Build history of the part. All positions in model axes, mm. Give positions to 0.01 mm unless a question says otherwise; leave off trailing zeros. Order: outer loops, then holes, each group sorted by start corner. A loop starts at its lowest first (then second) coordinate and runs counter-clockwise, first axis right, second up. Notation, with made-up numbers: (-36, 8) - (8, 8) arc R18 cw to (8, 24) - close; hole circle Ø7 at (-30.5, 39.5). An arc over 180 degrees is marked (long way). Use a Markdown table: item, result.
from build123d import *

# Parameters (mm, degrees)
F1_DEPTH = 2.15
F3_DEPTH = 3.1
F5_DEPTH = 0.8
F9_DEPTH = 1.4


with BuildPart() as f1:
    # F0 (on Top) → F1 (new body)
    with BuildSketch(Plane.XY):
        Polygon((-50.2594385356, -11.2599956296), (0, -11.2599956296), (0, 6.3900043704), (-47.2094385356, 6.3900043704), (-47.2094385356, 1.7900043704), (-47.9594385356, 1.7900043704), (-47.9594385356, 10.5400043704), (-50.2594385356, 10.5400043704), align=None)
        Polygon((0, 6.3900043704), (0, -11.2599956296), (50.2594385356, -11.2599956296), (50.2594385356, 10.5400043704), (47.9594385356, 10.5400043704), (47.9594385356, 1.7900043704), (47.2094385356, 1.7900043704), (47.2094385356, 6.3900043704), align=None)
    extrude(amount=F1_DEPTH)

    # F2 (on face) → F3 (join)
    with BuildSketch(Plane.XY.offset(2.15)):
        Polygon((-47.9594385356, -9.0099956296), (-47.9594385356, 1.7900043704), (-47.9594385356, 10.5400043704), (-50.2594385356, 10.5400043704), (-50.2594385356, -11.2599956296), (50.2594385356, -11.2599956296), (50.2594385356, 10.5400043704), (47.9594385356, 10.5400043704), (47.9594385356, 1.7900043704), (47.9594385356, -9.0099956296), (0, -9.0099956296), align=None)
    extrude(amount=F3_DEPTH)

    # F4 (on face) → F5 (cut)
    with BuildSketch(Plane.XY.offset(5.25)):
        with BuildLine():
            Line((-49.6594385356, -9.0099956296), (-49.6594385356, 7.0900043704))
            Line((-49.6594385356, 7.0900043704), (-47.9594385356, 7.0900043704))
            Line((-47.9594385356, 7.0900043704), (-47.9594385356, 10.5400043704))
            Line((-47.9594385356, 10.5400043704), (-50.2594385356, 10.5400043704))
            Line((-50.2594385356, 10.5400043704), (-50.2594385356, -11.2599956296))
            Line((-50.2594385356, -11.2599956296), (50.2594385356, -11.2599956296))
            Line((50.2594385356, -11.2599956296), (50.2594385356, 10.5400043704))
            Line((50.2594385356, 10.5400043704), (47.9594385356, 10.5400043704))
            Line((47.9594385356, 10.5400043704), (47.9594385356, 7.0900043704))
            Line((47.9594385356, 7.0900043704), (49.6594385356, 7.0900043704))
            Line((49.6594385356, 7.0900043704), (49.6594385356, -9.0099956296))
            ThreePointArc((49.6594385356, -9.0099956296), (49.1615200636, -10.2120771576), (47.9594385356, -10.7099956296))
            Line((47.9594385356, -10.7099956296), (0, -10.7099956296))
            Line((0, -10.7099956296), (-47.9594385356, -10.7099956296))
            ThreePointArc((-47.9594385356, -10.7099956296), (-49.1615200636, -10.2120771576), (-49.6594385356, -9.0099956296))
        make_face()
    extrude(amount=-F5_DEPTH, mode=Mode.SUBTRACT)

    # F8 (on plane+point) → F9 (join)
    with BuildSketch(Plane(origin=(0, -1.5099956296, 0), x_dir=(-1, 0, 0), z_dir=(0, 1, 0))):
        Polygon((47.2594385356, 6.1), (39.3594385356, 2.15), (47.9594385356, 2.15), (47.9594385356, 5.25), (47.2594385356, 5.25), align=None)
    extrude(amount=F9_DEPTH)

    # F10: F1 across plane


with BuildPart() as f1_1:
    add(f1.part)
    add(f1.part.mirror(Plane.YZ))


solid = f1_1.part
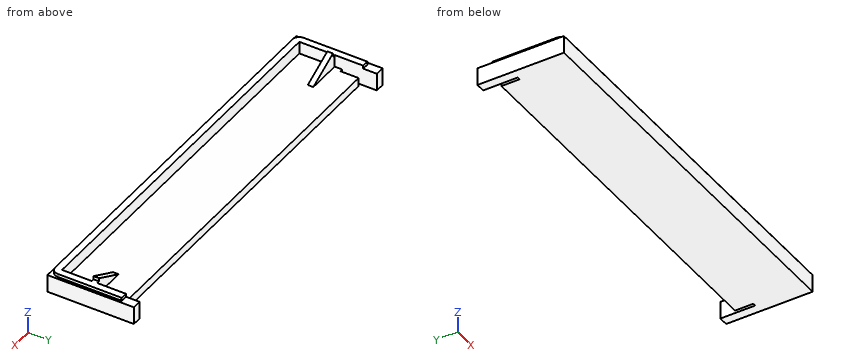
1) Slice it at D-D (y = -3.5). Write the cut outline in (x, z).
Computed:
| item | result |
|---|---|
| outline | (-50.26, 0) - (50.26, 0) - (50.26, 4.45) - (49.66, 4.45) - (49.66, 5.25) - (47.96, 5.25) - (47.96, 2.15) - (-47.96, 2.15) - (-47.96, 5.25) - (-49.66, 5.25) - (-49.66, 4.45) - (-50.26, 4.45) - close |
2) Pin check, flat tips, straight feed: P1, Ø1, axis at x = -7.5, z = 4.5, coming from the +Y side; P2, Ø11, axis at x = 9, y = -4, coming from the +Z side; P3, Ø0.9, axis at y = 2.5, z = 5, coming from the +X side. Stop position of each tip, or through.
Computed:
| item | result |
|---|---|
| P1 | stops at y = -9.01 |
| P2 | stops at z = 5.25 |
| P3 | stops at x = 49.66 |
3) Slice it at B-B (y = 3.5). Write the cut outline in (x, z), and give its area (3 significant figures).
Computed:
| item | result |
|---|---|
| outline | (-50.26, 0) - (-47.96, 0) - (-47.96, 5.25) - (-49.66, 5.25) - (-49.66, 4.45) - (-50.26, 4.45) - close; (-47.21, 0) - (47.21, 0) - (47.21, 2.15) - (-47.21, 2.15) - close; (47.96, 0) - (50.26, 0) - (50.26, 4.45) - (49.66, 4.45) - (49.66, 5.25) - (47.96, 5.25) - close |
| area | 226 mm² |
4) Slice it at C-C (x = 33). Write the cut outline in (y, z), and give its area (3 significant figures).
Computed:
| item | result |
|---|---|
| outline | (-11.26, 0) - (6.39, 0) - (6.39, 2.15) - (-9.01, 2.15) - (-9.01, 5.25) - (-10.71, 5.25) - (-10.71, 4.45) - (-11.26, 4.45) - close |
| area | 44.5 mm² |
5) Wall check: line 1 (X direction, y = 3, z = 0.5); line 2 (X direction, y = 5.25, z = 3.5); line 3 (Z direction, x = -12.5, y = 5.25). Give the ranges that are in metal, low to high. Write a range as from..to.
Computed:
| item | result |
|---|---|
| line 1 | x = -50.26..-47.96, -47.21..47.21, 47.96..50.26 |
| line 2 | x = -50.26..-47.96, 47.96..50.26 |
| line 3 | z = 0..2.15 |
6) Slice it at A-A (y = 9). Write the cut outline in (x, z).
Computed:
| item | result |
|---|---|
| outline | (-50.26, 0) - (-47.96, 0) - (-47.96, 4.45) - (-50.26, 4.45) - close; (47.96, 0) - (50.26, 0) - (50.26, 4.45) - (47.96, 4.45) - close |
